Here's how the part is built. I have some questions about the finished solid (model axes, mm). A direction names the side the tool comes from. Coordinates: 2 decimals unless noted, no trailing zeros. Write each loop counter-clockwise with the first axis right and the second up, starting at its lowest first coordinate (ties: lowest second). Pieces come first, ordered by that corner, then holes.
Item 1: I want a section at D-D (z = -8). Please give me the cut outline in (x, y), and give its area (3 significant figures).
Item 2: Please list where these lines run through material, in increasing order: line 1 (Y direction, x = 4.5, z = 6); line 2 (Y direction, x = 25, z = -4); line 3 (Z direction, x = 0, y = 18.2).
Item 3: I want a section at A-A (z = 14). Please give me the cut outline in (x, y).
Item 4: I'm going to push flat-ended pins straight in: P1, Ø10.5, axis at x = 0, z = 0, coming from the -Y side; P2, Ø3, axis at x = -1.5, y = -11, coming from the -Z side; P3, Ø0.9, axis at y = -38, z = 6.5, coming from the -X side. Where does each tip first touch, or does it pass through?
Item 5: I want a section at B-B (x = -10). Please give me the cut outline in (y, z) (3 decimals).
Item 6: I want a section at C-C (y = -44). Please give me the cut outline in (x, z) (3 decimals).
Item 7: If we mould it in two halves opening along X, with no side actions, what happens to faces 5 (the face through (0, -35, 17)), 6 (the face through (27.5, -7, 16)), 7 (the face through (22.16, 1.48, -0.19))? For each: pulls with the +X half, pulls with the -X half, needs draft (parallel to the pull), parting line crosses it, or undercut.
Item 8: For faces 1 (the face through (-6, -20, 3)), 2 (the face through (6, -46, 18)), 3 (the face through (0, 3, 9)), 4 (the face through (-3.955, -21.479, -5.158)), which set-ups out of +Z, -Z, +X, -X, +Y, -Y let a thin tool reach every point of the face, with its end or its side?
from build123d import *

# Parameters (mm, degrees)
SKETCH1_W                = 55
SKETCH1_H                = 32
SKETCH1_R                = 0.875
SKETCH1_R_2              = 6.5
BOSS_EXTRUDE1_DEPTH      = 3
BOSS_EXTRUDE2_START      = 3
SKETCH1_4_W              = 55
SKETCH1_4_H              = 5
BOSS_EXTRUDE2_DEPTH      = 13
BOSS_EXTRUDE3_START      = 16
BOSS_EXTRUDE3_DEPTH      = 3
BOSS_EXTRUDE4_START      = 19
BOSS_EXTRUDE4_DEPTH      = 15
SKETCH1_7_W              = 55
SKETCH1_7_H              = 5
BOSS_EXTRUDE5_DEPTH      = 10
SKETCH2_R                = 0.875
CUT_EXTRUDE1_DEPTH       = 52.393092921
CHAMFER1_SIZE            = 5
CHAMFER1_OF_MIRROR4_SIZE = 5
SKETCH3_W                = 5
SKETCH3_H                = 10
BOSS_EXTRUDE6_DEPTH      = 23


with BuildPart() as part:
    # Sketch1 → Boss-Extrude1 (new body)
    with BuildSketch(Plane(origin=(0, 0, 0), x_dir=(1, 0, 0), z_dir=(0, 1, 0))):
        with Locations((0, -6)):
            Rectangle(SKETCH1_W, SKETCH1_H)
        with Locations(Location((-23.0125, 0, 0), (0, 0, 270))):
            Circle(SKETCH1_R, mode=Mode.SUBTRACT)
        with Locations(Location((23.0125, 0, 0), (0, 0, 270))):
            Circle(SKETCH1_R, mode=Mode.SUBTRACT)
        with Locations(Location((0, 0, 0), (0, 0, 270))):
            Circle(SKETCH1_R_2, mode=Mode.SUBTRACT)
    boss_extrude1 = extrude(amount=BOSS_EXTRUDE1_DEPTH)

    # Sketch1<4> → Boss-Extrude2 (add)
    with BuildSketch(Plane(origin=(0, 0, 0), x_dir=(1, 0, 0), z_dir=(0, 1, 0)).offset(BOSS_EXTRUDE2_START)):
        with Locations((0, -19.5)):
            Rectangle(SKETCH1_4_W, SKETCH1_4_H)
    boss_extrude2 = extrude(amount=BOSS_EXTRUDE2_DEPTH)

    # Sketch1<5> → Boss-Extrude3 (add)
    with BuildSketch(Plane(origin=(0, 0, 0), x_dir=(1, 0, 0), z_dir=(0, 1, 0)).offset(BOSS_EXTRUDE3_START)):
        with BuildLine():
            Line((7, -17), (7, 0))
            Line((7, 0), (6.5, 0))
            ThreePointArc((6.5, 0), (0, -6.5), (-6.5, 0))
            Line((-6.5, 0), (-7, 0))
            Line((-7, 0), (-7, -17))
            Line((-7, -17), (-5, -17))
            Line((-5, -17), (5, -17))
            Line((5, -17), (7, -17))
        make_face()
        with BuildLine():
            ThreePointArc((-6.5, 0), (0, -6.5), (6.5, 0))
            Line((6.5, 0), (4.05, 0))
            ThreePointArc((4.05, 0), (0, -4.05), (-4.05, 0))
            Line((-4.05, 0), (-6.5, 0))
        make_face()
        with BuildLine():
            Line((4.05, 0), (6.5, 0))
            ThreePointArc((6.5, 0), (0, 6.5), (-6.5, 0))
            Line((-6.5, 0), (-4.05, 0))
            ThreePointArc((-4.05, 0), (0, 4.05), (4.05, 0))
        make_face()
        with BuildLine():
            Line((6.5, 0), (7, 0))
            ThreePointArc((7, 0), (0, 7), (-7, 0))
            Line((-7, 0), (-6.5, 0))
            ThreePointArc((-6.5, 0), (0, 6.5), (6.5, 0))
        make_face()
        Polygon((27.5, -17), (7, -17), (5, -17), (5, -18), (8, -18), (8, -20), (-8, -20), (-8, -18), (-5, -18), (-5, -17), (-7, -17), (-27.5, -17), (-27.5, -22), (27.5, -22), align=None)
        Polygon((5, -18), (5, -17), (-5, -17), (-5, -18), (-8, -18), (-8, -20), (8, -20), (8, -18), align=None)
    boss_extrude3 = extrude(amount=BOSS_EXTRUDE3_DEPTH)

    # Sketch1<6> → Boss-Extrude4 (add)
    with BuildSketch(Plane(origin=(0, 0, 0), x_dir=(1, 0, 0), z_dir=(0, 1, 0)).offset(BOSS_EXTRUDE4_START)):
        Polygon((-7, -17), (-27.5, -17), (-27.5, -22), (27.5, -22), (27.5, -17), (7, -17), (5, -17), (5, -18), (8, -18), (8, -20), (-8, -20), (-8, -18), (-5, -18), (-5, -17), align=None)
    boss_extrude4 = extrude(amount=BOSS_EXTRUDE4_DEPTH)

    # Sketch1<7> → Boss-Extrude5 (add)
    with BuildSketch(Plane(origin=(0, 0, 0), x_dir=(1, 0, 0), z_dir=(0, 1, 0))):
        with Locations((0, -19.5)):
            Rectangle(SKETCH1_7_W, SKETCH1_7_H)
    boss_extrude5 = extrude(amount=-BOSS_EXTRUDE5_DEPTH)

    # Sketch2 → Cut-Extrude1 (cut, through all)
    with BuildSketch(Plane(origin=(0, 0, 17), x_dir=(-1, 0, 0), z_dir=(0, 0, -1))):
        with Locations((-10, 24)):
            Circle(SKETCH2_R)
        with Locations((10, 24)):
            Circle(SKETCH2_R)
    cut_extrude1 = extrude(amount=-CUT_EXTRUDE1_DEPTH, mode=Mode.SUBTRACT)

    # Chamfer1
    chamfer1_edges = [part.edges().sort_by_distance(p)[0] for p in [
        (7, 17.5, 17),
        (-7, 17.5, 17),
    ]]
    chamfer(chamfer1_edges, length=CHAMFER1_SIZE)

    # Mirror4: Boss-Extrude1, Boss-Extrude2, Boss-Extrude3, Boss-Extrude4, Boss-Extrude5, Cut-Extrude1 across plane
    add(boss_extrude1.mirror(Plane(origin=(0, -10, 0), x_dir=(0, 0, 1), z_dir=(0, -1, 0))))
    add(boss_extrude2.mirror(Plane(origin=(0, -10, 0), x_dir=(0, 0, 1), z_dir=(0, -1, 0))))
    add(boss_extrude3.mirror(Plane(origin=(0, -10, 0), x_dir=(0, 0, 1), z_dir=(0, -1, 0))))
    add(boss_extrude4.mirror(Plane(origin=(0, -10, 0), x_dir=(0, 0, 1), z_dir=(0, -1, 0))))
    add(boss_extrude5.mirror(Plane(origin=(0, -10, 0), x_dir=(0, 0, 1), z_dir=(0, -1, 0))))
    add(cut_extrude1.mirror(Plane(origin=(0, -10, 0), x_dir=(0, 0, 1), z_dir=(0, -1, 0))), mode=Mode.SUBTRACT)

    # Chamfer1 of Mirror4
    chamfer1_of_mirror4_edges = [part.edges().sort_by_distance(p)[0] for p in [
        (7, -37.5, 17),
        (-7, -37.5, 17),
    ]]
    chamfer(chamfer1_of_mirror4_edges, length=CHAMFER1_OF_MIRROR4_SIZE)

    # Sketch3 → Boss-Extrude6 (add)
    with BuildSketch(Plane.XZ.offset(23)):
        with Locations((-25, 12)):
            Rectangle(SKETCH3_W, SKETCH3_H)
        with Locations((25, 12)):
            Rectangle(SKETCH3_W, SKETCH3_H)
    extrude(amount=-BOSS_EXTRUDE6_DEPTH)


solid = part.part
Answer:
1. outline: (-27.5, -23) - (27.5, -23) - (27.5, -20) - (-27.5, -20) - close; (-27.5, 0) - (27.5, 0) - (27.5, 3) - (-27.5, 3) - close
1. area: 330 mm2
2. line 1: y = -39 to -36, -23 to -20, 0 to 3, 16 to 19
2. line 2: y = -23 to -20, 0 to 3
2. line 3: z = -7 to -4.05, 4.05 to 22
3. outline: (-27.5, -23) - (27.5, -23) - (27.5, 3) - (-27.5, 3) - close; (-9, -39) - (9, -39) - (9, -36) - (-9, -36) - close; (-9, 16) - (9, 16) - (9, 19) - (-9, 19) - close; hole (-22.5, -20) - (22.5, -20) - (22.5, 0) - (-22.5, 0) - close
4. P1: stops at y = -39
4. P2: stops at z = 17
4. P3: stops at x = -7
5. outline: (-54, 17) - (-44.875, 17) - (-44.875, 22) - (-54, 22) - close; (-43.125, 17) - (-39, 17) - (-39, 15) - (-36, 15) - (-36, 17) - (-23, 17) - (-23, -10) - (-20, -10) - (-20, 17) - (0, 17) - (0, -10) - (3, -10) - (3, 17) - (16, 17) - (16, 15) - (19, 15) - (19, 17) - (23.125, 17) - (23.125, 22) - (-43.125, 22) - close; (24.875, 17) - (34, 17) - (34, 22) - (24.875, 22) - close
6. outline: (-27.5, 17) - (-10.875, 17) - (-10.875, 22) - (-27.5, 22) - close; (-9.125, 17) - (-5, 17) - (-5, 18) - (-8, 18) - (-8, 20) - (8, 20) - (8, 18) - (5, 18) - (5, 17) - (9.125, 17) - (9.125, 22) - (-9.125, 22) - close; (10.875, 17) - (27.5, 17) - (27.5, 22) - (10.875, 22) - close
7. face 5: needs draft
7. face 6: pulls with the +X half
7. face 7: undercut
8. face 1: -Z
8. face 2: -Y
8. face 3: -Z, +X, -X
8. face 4: none
